Check sheet for the modelled part. Datum: model origin and axes. Units: mm. Face numbers are marked on the shaded views. A direction names the side the tool comes from. Coordinates: 2 decimals unless noted, no trailing zeros. Loops run counter-clockwise (first coordinate to the right, second up) from the corner with the lowest first, then second, coordinate; pieces in that order, holes last. Notation, with made-up numbers: M -25.5,88 L 22.5,88 A17 ccw 22.5,100 Z; hole C -29.75,62.5 d2. An arc over 180 degrees is marked long. Answer in a Markdown table with one row per item. Add a question column.
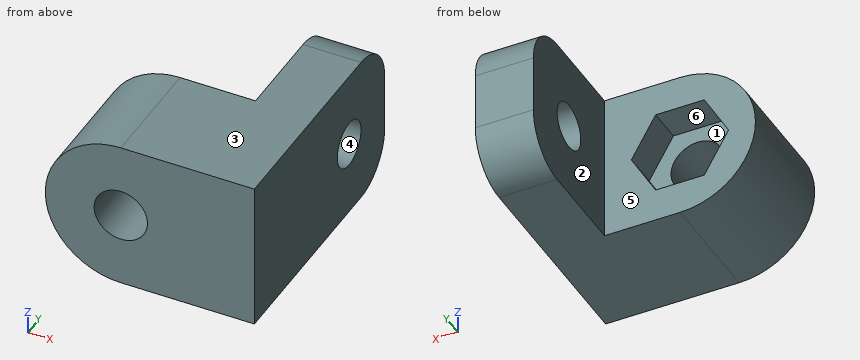
Autodesk Inventor part; units mm, degrees
ref_plane "Work Plane1" through (6.5, 0, 0) normal (1, 0, 0) x (0, 1, 0)
ref_plane "XZ Plane" through (0, 0, 0) normal (0, 1, 0) x (-1, 0, 0)
ref_plane "XY Plane" through (0, 0, 0) normal (0, 0, 1) x (1, 0, 0)
sketch "Sketch1" plane through (0, 0, 0) normal (0, 1, 0) x (-1, 0, 0)
  circle A0 centre (0, 0) radius 6.5
  circle A1 centre (0, 0) radius 2.3
  dimension "d0" = 13
  dimension "d1" = 4.6
extrude "Extrusion1" add sketch "Sketch1" along normal blind 10
sketch "Sketch2" plane through (0, 10, 0) normal (0, 1, 0) x (1, 0, 0)
  point P0 (0, 0)
ref_plane "Work Plane1" through (6.5, 0, 0) normal (1, 0, 0) x (0, 1, 0)
sketch "Sketch3" plane through (6.5, 0, 0) normal (1, 0, 0) x (0, 1, 0)
  line L0 (10, -6.5) -> (10, 6.5)
  line L1 (10, -6.5) -> (22, -6.5)
  line L2 (22, -6.5) -> (22, 6.5)
  line L3 (22, 6.5) -> (10, 6.5)
  line L4 (10, 6.5) -> (10, -6.5)
  line L5 (0, -6.5) -> (0, 6.5)
  line L6 (10, -6.5) -> (0, -6.5)
  line L7 (0, -6.5) -> (0, 6.5)
  line L8 (0, 6.5) -> (10, 6.5)
  line L9 (10, 6.5) -> (10, -6.5)
  circle A0 centre (16, 0) radius 2
  point P0 (0, 0)
  point P1 (0, -6.5)
  point P2 (10, 6.5)
  point P3 (10, 6.5)
  dimension "d5" = 12
  dimension "d6" = 4
  dimension "d11" = 6
extrude "Extrusion2" add sketch "Sketch3" against normal up to surface contours L6 L5 L8 L0
extrude "Extrusion3" add sketch "Sketch3" along normal blind 5
sketch "Sketch5" plane through (0, 10, 0) normal (0, 1, 0) x (1, 0, 0)
  line L0 (4.1858, 0) -> (2.0929, -3.625)
  line L1 (2.0929, -3.625) -> (-2.0929, -3.625)
  line L2 (-2.0929, -3.625) -> (-4.1858, 0)
  line L3 (-4.1858, 0) -> (-2.0929, 3.625)
  line L4 (-2.0929, 3.625) -> (2.0929, 3.625)
  line L5 (2.0929, 3.625) -> (4.1858, 0)
  point P0 (0, 0)
  point P1 (0, 0)
  dimension "d12" = 7.25
extrude "Extrusion4" cut sketch "Sketch5" against normal blind 3
fillet "Fillet1" radius 4 2 edges at (9, 22, 6.5) (9, 22, -6.5)
properties part number "SpringConn"
Q1. Thickness scan on L1, parallel to X at y = 2.5, z = 0; L2, parallel to Z at x = 9.7, y = 16; L3, parallel to Y at x = -4, z = 4.5. Record the ranges inside material, lowest first.
Q2. Access from +Z, -Z, +X, -X, +Y, -Y to the whole of each face (thin tool, end or side, straight path). Record for the marked faces 4, 5 and 6.
Q3. Cross-section at B-B (x = 1). Record the cut outline in (y, z) (3 decimals).
Q4. Cross-section at C-C (z = -1). Record the cut outline in (x, y), plus the area to 3 significant figures.
Q5. Go/stop test with a flat-tipped pin: pin 1 (6 mm diameter, centred on y = 16.5, z = -1.5, fed in from -X). Record where the tip stops, or that it passes through.
Q6. Cross-section at A-A (y = 16). Record the cut outline in (x, z), plus the area to 3 significant figures.
Q7. Cross-section at D-D (y = 5.75). Record the cut outline in (x, z).
Q8. Mould release check, pull along Z, two halves, no side actions. Record for the marked faces 1, 2 and 3: released by +Z, released by -Z, zero draft, split by the parting line, or undercut.
Answer key:
| question | item | result |
|---|---|---|
| 1 | L1 | -6.5 to -2.3, 2.3 to 11.5 |
| 1 | L2 | -6.5 to -2, 2 to 6.5 |
| 1 | L3 | 0 to 10 |
| 2 | face 4 | +X, -X |
| 2 | face 5 | +Z, -Z, -X, +Y |
| 2 | face 6 | +Y |
| 3 | outline | M 0,-6.5 L 10,-6.5 L 10,-3.625 L 7,-3.625 L 7,-2.071 L 0,-2.071 Z; M 0,2.071 L 7,2.071 L 7,3.625 L 10,3.625 L 10,6.5 L 0,6.5 Z |
| 4 | outline | M -6.42,0 L -2.07,0 L -2.07,7 L -3.61,7 L -3.61,10 L -6.42,10 Z; M 2.07,0 L 11.5,0 L 11.5,14.27 L 6.5,14.27 L 6.5,10 L 3.61,10 L 3.61,7 L 2.07,7 Z; M 6.5,17.73 L 11.5,17.73 L 11.5,22 L 6.5,22 Z |
| 4 | area | 171 mm^2 |
| 5 | pin 1 | x = 6.5 |
| 6 | outline | M 6.5,-6.5 L 11.5,-6.5 L 11.5,-2 L 6.5,-2 Z; M 6.5,2 L 11.5,2 L 11.5,6.5 L 6.5,6.5 Z |
| 6 | area | 45.0 mm^2 |
| 7 | outline | M 0,-6.5 L 11.5,-6.5 L 11.5,6.5 L 0,6.5 A6.5 ccw Z; hole C 0,0 d4.6 |
| 8 | face 1 | undercut |
| 8 | face 2 | zero draft |
| 8 | face 3 | released by +Z |
